Autodesk Inventor part; units mm, degrees
ref_plane "YZ Plane" through (0, 0, 0) normal (1, 0, 0) x (0, 1, 0)
ref_plane "XZ Plane" through (0, 0, 0) normal (0, 1, 0) x (-1, 0, 0)
ref_plane "XY Plane" through (0, 0, 0) normal (0, 0, 1) x (1, 0, 0)
sketch "Sketch1" plane through (0, 0, 0) normal (0, 0, 1) x (1, 0, 0)
  circle A0 centre (-219.1094, -175.8797) radius 11.5
  circle A1 centre (219.1094, -175.8797) radius 11.5
  line L0 (264.1156, -220.8859) -> (-264.1156, -220.8859)
  line L1 (264.1156, 220.8859) -> (264.1156, -220.8859)
  line L2 (-264.1156, 220.8859) -> (264.1156, 220.8859)
  line L3 (-264.1156, -220.8859) -> (-264.1156, 220.8859)
  line L4 (200, 196.1016) -> (-200, 196.1016)
  line L5 (200, -131.8984) -> (200, 196.1016)
  line L6 (-200, -131.8984) -> (200, -131.8984)
  line L7 (-200, 196.1016) -> (-200, -131.8984)
  line L8 (139, 202.1016) -> (119, 202.1016)
  line L9 (206, 187.0016) -> (206, 167.0016)
  line L10 (-206, 187.0016) -> (-206, 167.0016)
  line L11 (-206, -102.7984) -> (-206, -122.7984)
  line L12 (206, -122.7984) -> (206, -102.7984)
  line L13 (-206, 202.1016) -> (206, 202.1016)
  line L14 (206, 202.1016) -> (206, -131.8984)
  line L15 (206, -131.8984) -> (-206, -131.8984)
  line L16 (-206, -131.8984) -> (-206, 202.1016)
  line L17 (207, 203.1016) -> (-207, 203.1016)
  line L18 (-207, 203.1016) -> (-207, -132.8984)
  line L19 (-207, -132.8984) -> (207, -132.8984)
  line L20 (207, -132.8984) -> (207, 203.1016)
  circle A2 centre (219.1094, -175.8797) radius 9.5
  circle A3 centre (-219.1094, -175.8797) radius 9.5
  circle A4 centre (-219.1094, -175.8797) radius 11.5
  circle A5 centre (-219.1094, -175.8797) radius 11.5
  circle A6 centre (-219.1094, -175.8797) radius 11.5
  point P0 (0, 0)
  dimension "d0" = 1
extrude "Extrusion1" add sketch "Sketch1" along normal blind 12 contours A0 | A1 | L0 L3 L2 L1
sketch "Sketch2" plane through (0, 0, 0) normal (0, 0, -1) x (-1, 0, 0)
  line L0 (0, 210.8859) -> (254.1156, 210.8859) construction
  line L1 (254.1156, 210.8859) -> (254.1156, 0) construction
  line L2 (254.1156, 0) -> (0, 0) construction
  line L3 (0, 0) -> (0, 210.8859) construction
  line L4 (-264.1156, 220.8859) -> (264.1156, 220.8859) construction
  line L5 (264.1156, 220.8859) -> (264.1156, -220.8859) construction
  point P0 (127.0578, 210.8859)
  point P1 (254.1156, 114.7989)
  dimension "d3" = 10
  dimension "d4" = 10
hole "Hole1" at (0, 210.8859, 0) at (-127.0578, 210.8859, 0) at (-254.1156, 210.8859, 0) at (-254.1156, 114.7989, 0) at (-254.1156, 0, 0) direction (0, 0, 1) diameter 2 end through all
mirror "Mirror1" about plane through (0, 0, 0) normal (1, 0, 0) of "Hole1"
mirror "Mirror2" about plane through (0, 0, 0) normal (0, 1, 0) of "Hole1", "Mirror1"
properties part number "lag3"
Verification items for the finished model (mm, model axes). A direction names the side the tool comes from. Give positions to 0.01 mm unless a question says otherwise; leave off trailing zeros. Order: outer loops, then holes, each group sorted by start corner. A loop starts at its lowest first (then second) coordinate and runs counter-clockwise, first axis right, second up. Notation, with made-up numbers: M -27,49 L 29,49 A8 cw 29,61 Z; hole C -16,43 d11. An arc over 180 degrees is marked long. Use one line per item in the form item = value. Start each with the question number.
Q1. Access from +Z, -Z, +X, -X, +Y, -Y to the whole of each face (thin tool, end or side, straight path). Record for faces 5 (the flat face through (-207, 37, 6)), 6 (the flat face through (-264.116, -3, 6)).
Q2. Section check B-B (x = -24). Enter the section's corners in (y, z).
Q3. Scan lines: line 1 along X through (y, z) = (0, 8.75); line 2 along Y through (x, z) = (-77.5, 10.5); line 3 along X through (y, z) = (142.5, 3.5). Record each from-to range of solid material in increasing order. Write a range as [from, to].
Q4. Mould release check, pull along Y, two halves, no side actions. Record for faces 1 (the flat face through (-4, -144, 0)), 2 (the flat face through (3, 203.102, 6)), 3 (the flat face through (4, -220.886, 6)), 4 (the flat face through (-4, 220.886, 6)): +Y half, -Y half, draft (parallel to the pull), parting line (faces both ways), or undercut.
Q5. Section check C-C (z = 5.5). Count the separate pieces of the cut face and the enclosed holes in it, then the cut area to 3 significant figures.
Q6. Section check A-A (y = 22). Enter the section's corners in (x, z).
Evaluation:
q1.face_5 = +Z, -Z
q1.face_6 = +Z, -Z, -X, +Y, -Y
q2.outline = M -220.89,0 L -132.9,0 L -132.9,12 L -220.89,12 Z; M 203.1,0 L 220.89,0 L 220.89,12 L 203.1,12 Z
q3.line_1 = [-264.12, -255.12], [-253.12, -207], [207, 253.12], [255.12, 264.12]
q3.line_2 = [-220.89, -132.9], [203.1, 220.89]
q3.line_3 = [-264.12, -207], [207, 264.12]
q4.face_1 = draft
q4.face_2 = undercut
q4.face_3 = -Y half
q4.face_4 = +Y half
q5.separate_pieces = 1
q5.enclosed_holes = 19
q5.area = 93,600 mm2
q6.outline = M -264.12,0 L -207,0 L -207,12 L -264.12,12 Z; M 207,0 L 264.12,0 L 264.12,12 L 207,12 Z
